```python
from build123d import *

# Parameters (mm, degrees)
SKETCH_1_W           = 80
SKETCH_1_H           = 156.363783163
EXTRUDE_1_DEPTH      = 90
SKETCH_3_W           = 30
SKETCH_3_H           = 30
CUT_EXTRUDE_1_DEPTH  = 15
SKETCH_4_W           = 182.158516052
SKETCH_4_H           = 121.356957168
CUT_EXTRUDE_2_DEPTH  = 60
SKETCH_6_W           = 50.175493085
SKETCH_6_H           = 149.046749465
CUT_EXTRUDE_4_DEPTH  = 16
SKETCH_7_W           = 13.065428471
SKETCH_7_H           = 30
CUT_EXTRUDE_5_DEPTH  = 147.711160425
SKETCH_8_W           = 28.25361391
SKETCH_8_H           = 169.077909422
CUT_EXTRUDE_6_DEPTH  = 85
SKETCH_10_W          = 25
SKETCH_10_H          = 25
CUT_EXTRUDE_7_DEPTH  = 5
SKETCH_11_W          = 25
SKETCH_11_H          = 7.062774738
CUT_EXTRUDE_8_DEPTH  = 133.850158424
SKETCH_12_R          = 1.553167794
CUT_EXTRUDE_9_DEPTH  = 144.698171851
FILLET_3_R           = 10
CUT_EXTRUDE_START    = 60
SKETCH_15_W          = 25.147195628
SKETCH_15_H          = 171.888478346
CUT_EXTRUDE_10_DEPTH = 85
FILLET_6_R           = 10
FILLET_7_R           = 10
SKETCH_18_W          = 152.348651532
SKETCH_18_H          = 32.578688912
CUT_EXTRUDE_11_DEPTH = 147.711160425
SKETCH_19_R          = 37.254412131
SKETCH_19_R_2        = 32.5
EXTRUDE_3_DEPTH      = 15
SKETCH_20_W          = 127.729938291
SKETCH_20_H          = 42.54840274
CUT_EXTRUDE_12_DEPTH = 185.159311294
EXTRUDE_5_DEPTH      = 15
EXTRUDE_START        = 15
EXTRUDE_6_DEPTH      = 15
EXTRUDE_7_DEPTH      = 15
SKETCH_27_R          = 1.5
CUT_EXTRUDE_13_DEPTH = 10


with BuildPart() as part:
    # 草图1 → 凸台-拉伸1 (new body)
    with BuildSketch(Plane.XY):
        with Locations((-9.441340782, -26.602259963)):
            Rectangle(SKETCH_1_W, SKETCH_1_H)
    extrude(amount=EXTRUDE_1_DEPTH)

    # 草图3 → 切除-拉伸1 (cut)
    with BuildSketch(Plane.XY.offset(90)):
        with Locations((-15.348450006, 27.268684522)):
            Rectangle(SKETCH_3_W, SKETCH_3_H)
    extrude(amount=-CUT_EXTRUDE_1_DEPTH, mode=Mode.SUBTRACT)

    # 草图4 → 切除-拉伸2 (cut)
    with BuildSketch(Plane.XY.offset(90)):
        with Locations((0, -58.480028538)):
            Rectangle(SKETCH_4_W, SKETCH_4_H)
    extrude(amount=-CUT_EXTRUDE_2_DEPTH, mode=Mode.SUBTRACT)

    # 草图6 → 切除-拉伸4 (cut)
    with BuildSketch(Plane(origin=(0, 0, 0), x_dir=(-1, 0, 0), z_dir=(0, 0, -1))):
        with Locations((9.964306437, -36.113761051)):
            Rectangle(SKETCH_6_W, SKETCH_6_H)
    extrude(amount=-CUT_EXTRUDE_4_DEPTH, mode=Mode.SUBTRACT)

    # 草图7 → 切除-拉伸5 (cut, through all)
    with BuildSketch(Plane.XY.offset(90)):
        with Locations((6.18426423, 27.268684522)):
            Rectangle(SKETCH_7_W, SKETCH_7_H)
    extrude(amount=-CUT_EXTRUDE_5_DEPTH, mode=Mode.SUBTRACT)

    # 草图8 → 切除-拉伸6 (cut)
    with BuildSketch(Plane.XY.offset(90)):
        with Locations((-55.342514846, -28.081506765)):
            Rectangle(SKETCH_8_W, SKETCH_8_H)
    extrude(amount=-CUT_EXTRUDE_6_DEPTH, mode=Mode.SUBTRACT)

    # 草图10 → 切除-拉伸7 (cut)
    with BuildSketch(Plane.XY.offset(30)):
        with Locations((-9.930002564, -33.110581364)):
            Rectangle(SKETCH_10_W, SKETCH_10_H)
    extrude(amount=-CUT_EXTRUDE_7_DEPTH, mode=Mode.SUBTRACT)

    # 草图11 → 切除-拉伸8 (cut, through all)
    with BuildSketch(Plane.XY.offset(25)):
        with Locations((-9.930002564, -42.079193995)):
            Rectangle(SKETCH_11_W, SKETCH_11_H)
    extrude(amount=-CUT_EXTRUDE_8_DEPTH, mode=Mode.SUBTRACT)

    # 草图12 → 切除-拉伸9 (cut, through all)
    with BuildSketch(Plane.XY.offset(5)):
        with Locations((-45.941340782, 41.579631618)):
            Circle(SKETCH_12_R)
        with Locations((27.058659218, 41.579631618)):
            Circle(SKETCH_12_R)
        with Locations((-45.941340782, 11.579631618)):
            Circle(SKETCH_12_R)
        with Locations((-45.941340782, -28.420368382)):
            Circle(SKETCH_12_R)
        with Locations((27.058659218, 11.579631618)):
            Circle(SKETCH_12_R)
        with Locations((27.058659218, -28.420368382)):
            Circle(SKETCH_12_R)
        with Locations((-45.941340782, -58.420368382)):
            Circle(SKETCH_12_R)
        with Locations((27.058659218, -58.420368382)):
            Circle(SKETCH_12_R)
    extrude(amount=-CUT_EXTRUDE_9_DEPTH, mode=Mode.SUBTRACT)

    # 圆角3
    fillet_3_edges = [part.edges().sort_by_distance(p)[0] for p in [
        (-41.215707891, -51.292850749, 30),
    ]]
    fillet(fillet_3_edges, radius=FILLET_3_R)

    # 草图15 → 切除-拉伸10 (cut)
    with BuildSketch(Plane.XY.offset(30).offset(CUT_EXTRUDE_START)):
        with Locations((34.196439865, -22.534331259)):
            Rectangle(SKETCH_15_W, SKETCH_15_H)
    extrude(amount=-CUT_EXTRUDE_10_DEPTH, mode=Mode.SUBTRACT)

    # 圆角6
    fillet_6_edges = [part.edges().sort_by_distance(p)[0] for p in [
        (21.622842051, -51.292850749, 30),
    ]]
    fillet(fillet_6_edges, radius=FILLET_6_R)

    # 圆角7
    fillet_7_edges = [part.edges().sort_by_distance(p)[0] for p in [
        (21.622842051, 2.198450046, 55),
        (-41.215707891, 2.198450046, 55),
        (-41.215707891, 51.579631618, 47.5),
        (21.622842051, 51.579631618, 47.5),
    ]]
    fillet(fillet_7_edges, radius=FILLET_7_R)

    # 草图18 → 切除-拉伸11 (cut, through all)
    with BuildSketch(Plane(origin=(0, 0, 0), x_dir=(-1, 0, 0), z_dir=(0, 0, -1))):
        with Locations((19.986133812, -102.5828817)):
            Rectangle(SKETCH_18_W, SKETCH_18_H)
    extrude(amount=-CUT_EXTRUDE_11_DEPTH, mode=Mode.SUBTRACT)

    # 草图19 → 凸台-拉伸3 (add)
    with BuildSketch(Plane.XZ.offset(86.293537244)):
        with Locations(Location((-9.79643292, 0, 0), (0, 0, 126.427336474))):
            Circle(SKETCH_19_R)
        with Locations(Location((-9.79643292, 0, 0), (0, 0, 112.619864948))):
            Circle(SKETCH_19_R_2, mode=Mode.SUBTRACT)
    extrude(amount=EXTRUDE_3_DEPTH)

    # 草图20 → 切除-拉伸12 (cut, through all)
    with BuildSketch(Plane.XZ.offset(101.293537244)):
        with Locations((-5.047238287, -21.27420137)):
            Rectangle(SKETCH_20_W, SKETCH_20_H)
    extrude(amount=-CUT_EXTRUDE_12_DEPTH, mode=Mode.SUBTRACT)

    # 草图24 → 凸台-拉伸5 (add)
    with BuildSketch(Plane(origin=(0, -86.293537244, 0), x_dir=(1, 0, 0), z_dir=(0, 1, 0))):
        with BuildLine():
            Line((-46.713789586, -5), (-41.215707891, -5))
            Line((-41.215707891, -5), (-41.215707891, -20))
            ThreePointArc((-41.215707891, -20), (-44.727814177, -12.779693075), (-46.713789586, -5))
        make_face()
    extrude(amount=EXTRUDE_5_DEPTH)

    # 草图25 → 凸台-拉伸6 (add)
    with BuildSketch(Plane(origin=(0, -86.293537244, 0), x_dir=(1, 0, 0), z_dir=(0, 1, 0)).offset(EXTRUDE_START)):
        with BuildLine():
            Line((-31.918208762, -29.975294107), (12.325342922, -29.975294107))
            ThreePointArc((12.325342922, -29.975294107), (-9.79643292, -37.254412131), (-31.918208762, -29.975294107))
        make_face()
    extrude(amount=-EXTRUDE_6_DEPTH)

    # 草图26 → 凸台-拉伸7 (add)
    with BuildSketch(Plane(origin=(0, -86.293537244, 0), x_dir=(1, 0, 0), z_dir=(0, 1, 0))):
        with BuildLine():
            Line((27.120923747, -5), (21.622842051, -5))
            Line((21.622842051, -5), (21.622842051, -20))
            ThreePointArc((21.622842051, -20), (25.233426536, -12.815789153), (27.120923747, -5))
        make_face()
    extrude(amount=EXTRUDE_7_DEPTH)

    # 草图27 → 切除-拉伸13 (cut)
    with BuildSketch(Plane.XY.offset(25)):
        with Locations((-4.675690362, -23.954796266)):
            Circle(SKETCH_27_R)
        with Locations((-14.675690362, -23.954796266)):
            Circle(SKETCH_27_R)
    extrude(amount=-CUT_EXTRUDE_13_DEPTH, mode=Mode.SUBTRACT)


solid = part.part
```
Check sheet for the modelled part. Datum: model origin and axes. Units: mm. A direction names the side the tool comes from. Coordinates: 2 decimals unless noted, no trailing zeros. Order: outer loops, then holes, each group sorted by start corner. A loop starts at its lowest first (then second) coordinate and runs counter-clockwise, first axis right, second up. Notation, with made-up numbers: (-28.75, -32.5) -> (19.25, -32.5) arc R16 cw to (19.25, -10.5) -> close; hole circle Ø6 at (70.5, 59). An arc over 180 degrees is marked (long way). Write item = value, one per line. Start each with the question number.
1) Cross-section at D-D (z = 28). Enter the section's corners in (x, y).
2) Cross-section at C-C (y = -35.5). Enter the section's corners in (x, z).
3) Access from +Z, -Z, +X, -X, +Y, -Y to the whole of each face (thin tool, end or side, straight path). Record for faces 4 (the flat face through (-10, -20.611, 28)), 5 (the flat face through (21.623, 9.4, 19.8)), 6 (the flat face through (-10, -38.548, 21)).
4) Cross-section at A-A (z = 63). Enter the section's corners in (x, y), then the cut area to 3 significant figures.
5) Material ranges on L1, parallel to Y at x = -22, z = 19.5; L2, parallel to X at y = -3, z = 12; L3, parallel to Y at x = -6, z = 23, recorded low to high.
6) Cross-section at B-B (x = 5.5). Enter the section's corners in (y, z).
7) Mould release check, pull along Y, two halves, no side actions. Record for faces 1 (the flat face through (18, -86.294, 26)), 2 (the cylindrical face through (25.83, 10.63, 2.54)), 3 (the flat face through (30.559, -18, 2)): +Y half, -Y half, draft (parallel to the pull), parting line (faces both ways), or undercut.
8) Go/stop test with flat-tipped pins: P1, Ø15.5, axis at y = -38, z = 26, coming from the +X side; P2, Ø5, axis at x = 11, z = 21, coming from the -Y side; P3, Ø1.6, axis at x = 24, z = 11.5, coming from the +Y side; P4, Ø2.5, axis at x = 27.06, y = -58.42, coming from the -Z side. Record where each tip stops, or that it passes through.
Ans:
q1.outline = (-41.22, 12.2) arc R10 ccw to (-37.22, 4.2) -> (-37.22, -86.29) -> (-34.37, -86.29) -> (-34.37, -101.29) -> (-26.3, -101.29) -> (-26.3, -86.29) -> (6.7, -86.29) -> (6.7, -101.29) -> (14.78, -101.29) -> (14.78, -86.29) -> (17.62, -86.29) -> (17.62, 4.2) arc R10 ccw to (21.62, 12.2) -> (21.62, 41.58) arc R10 ccw to (11.62, 51.58) -> (-31.22, 51.58) arc R10 ccw to (-41.22, 41.58) -> close; hole (-22.43, -45.61) -> (2.57, -45.61) -> (2.57, -20.61) -> (-22.43, -20.61) -> close; hole (-0.35, 12.27) -> (12.72, 12.27) -> (12.72, 42.27) -> (-0.35, 42.27) -> close
q2.outline = (-49.44, 0) -> (-35.05, 0) -> (-35.05, 16) -> (15.12, 16) -> (15.12, 0) -> (30.56, 0) -> (30.56, 5) -> (21.62, 5) -> (21.62, 20) arc R10 ccw to (11.62, 30) -> (2.57, 30) -> (2.57, 25) -> (-22.43, 25) -> (-22.43, 30) -> (-31.22, 30) arc R10 ccw to (-41.22, 20) -> (-41.22, 5) -> (-49.44, 5) -> close
q3.face_4 = +Z
q3.face_5 = +Z, +X, +Y
q3.face_6 = +Z, -Z
q4.outline = (-41.22, 12.2) arc R10 ccw to (-31.22, 2.2) -> (11.62, 2.2) arc R10 ccw to (21.62, 12.2) -> (21.62, 41.58) arc R10 ccw to (11.62, 51.58) -> (-31.22, 51.58) arc R10 ccw to (-41.22, 41.58) -> close; hole (-0.35, 12.27) -> (12.72, 12.27) -> (12.72, 42.27) -> (-0.35, 42.27) -> close
q4.area = 2,630 mm²
q5.L1 = -86.29 to -45.61, -38.55 to 51.58
q5.L2 = -41.22 to -35.05, 15.12 to 21.62
q5.L3 = -86.29 to -45.61, -38.55 to -24.66, -23.25 to 51.58
q6.outline = (-101.29, 28.68) -> (-86.29, 28.68) -> (-86.29, 16) -> (12.27, 16) -> (12.27, 90) -> (2.2, 90) -> (2.2, 30) -> (-71.29, 30) -> (-71.29, 33.97) -> (-101.29, 33.97) -> close; (42.27, 0) -> (51.58, 0) -> (51.58, 90) -> (42.27, 90) -> close
q7.face_1 = -Y half
q7.face_2 = undercut
q7.face_3 = draft
q8.P1 = 21.62
q8.P2 = -86.29
q8.P3 = -71.29
q8.P4 = through
